```python
from build123d import *

# Parameters (mm, degrees)
F0_W           = 75
F0_H           = 50
F0_R           = 7.6
F1_DEPTH       = 4
F2_D           = 2.4
F3_D           = 3.2
F3_CSINK_D     = 6.72
F3_CSINK_ANGLE = 90
F4_R           = 7.5
F5_R           = 2.5


# Not quite as in the source:
# - a feature names something its author has since deleted; it is built from what else it names


with BuildPart() as f1:
    # F0 (on Top) → F1 (new body)
    with BuildSketch(Plane.XY):
        with Locations((0, 15)):
            Rectangle(F0_W, F0_H)
        Circle(F0_R, mode=Mode.SUBTRACT)
    extrude(amount=-F1_DEPTH)

    # F2 (through all)
    with Locations(Plane.XY):
        with Locations((-8, 8), (8, 8), (8, -8), (-8, -8)):
            Hole(F2_D / 2)

    # F3 (through all)
    with Locations(Plane.XY):
        with Locations((-25, 5), (25, 5), (-5, 28.5), (5, 28.5), (5, 13.5), (-5, 13.5), (-25, 35), (25, 35)):
            CounterSinkHole(F3_D / 2, F3_CSINK_D / 2, counter_sink_angle=F3_CSINK_ANGLE)

    # F4
    f4_edges = [f1.edges().sort_by_distance(p)[0] for p in [
        (-37.5, 40, -2),
        (37.5, 40, -2),
    ]]
    fillet(f4_edges, radius=F4_R)

    # F5
    f5_edges = [f1.edges().sort_by_distance(p)[0] for p in [
        (-37.5, -10, -2),
        (37.5, -10, -2),
    ]]
    fillet(f5_edges, radius=F5_R)


solid = f1.part
```
Can you work these out from the model? Positions are in its coordinate system, mm. Coordinates: 2 decimals unless noted, no trailing zeros. Loops run counter-clockwise (first coordinate to the right, second up) from the corner with the lowest first, then second, coordinate; pieces in that order, holes last. Notation, with made-up numbers: (75.5, 58) -> (119.5, 58) arc R24 ccw to (119.5, 90) -> close; hole circle Ø7 at (15.25, 61). An arc over 180 degrees is marked (long way). Put each result on its own line as item: value. Start each with the question number.
Q1. If I drill on line 1 (Y direction, x = -25, z = -2.55); line 2 (Y direction, x = -8, z = -1.25); line 3 (Y direction, x = -5, z = -2.55), over which ranges is the centre line in solid material (lowest first)? Write a range as [from, to].
Q2. I want a section at C-C (x = 25). Write out the boundary of the cut face in (y, z).
Q3. I want a section at A-A (y = 0). Write out the boundary of the cut face in (x, z).
Q4. I want a section at B-B (z = -2.65). Count the separate pieces of the cut face and the enclosed holes in it, plus the area to 3 significant figures.
Q5. I'm going to push flat-ended pins straight in: P1, Ø1.9, axis at x = 8, y = -8, coming from the +Z side; P2, Ø5, axis at x = -25, y = 35, coming from the +Z side; P3, Ø4, axis at x = 25, y = 35, coming from the +Z side. Where does each tip first touch, or does it pass through?
Q6. I want a section at D-D (y = 28.5). Write out the boundary of the cut face in (x, z).
Q7. Thinking about a two-plate mould opening in Y: for faces 1 (the face through (-35.361, 37.745, -2.028)), 2 (the face through (-4.792, 15.086, -2.896)), 3 (the face through (37.5, 12, -2)), which applies, pulls with the +Y half, pulls with the -Y half, needs draft (parallel to the pull), parting line crosses it, or undercut?
Taken from the geometry:
1. line 1: y = [-10, 3.4], [6.6, 33.4], [36.6, 40]
1. line 2: y = [-10, -9.2], [-6.8, 6.8], [9.2, 40]
1. line 3: y = [-10, -5.72], [5.72, 11.9], [15.1, 26.9], [30.1, 40]
2. outline: (-10, -4) -> (3.4, -4) -> (3.4, -1.76) -> (1.64, 0) -> (-10, 0) -> close; (6.6, -4) -> (33.4, -4) -> (33.4, -1.76) -> (31.64, 0) -> (8.36, 0) -> (6.6, -1.76) -> close; (36.6, -4) -> (40, -4) -> (40, 0) -> (38.36, 0) -> (36.6, -1.76) -> close
3. outline: (-37.5, -4) -> (-7.6, -4) -> (-7.6, 0) -> (-37.5, 0) -> close; (7.6, -4) -> (37.5, -4) -> (37.5, 0) -> (7.6, 0) -> close
4. separate pieces: 1
4. enclosed holes: 13
4. area: 3,460 mm2
5. P1: passes through
5. P2: stops at z = -0.86
5. P3: stops at z = -1.36
6. outline: (-37.5, -4) -> (-6.6, -4) -> (-6.6, -1.76) -> (-8.36, 0) -> (-37.5, 0) -> close; (-3.4, -4) -> (3.4, -4) -> (3.4, -1.76) -> (1.64, 0) -> (-1.64, 0) -> (-3.4, -1.76) -> close; (6.6, -4) -> (37.5, -4) -> (37.5, 0) -> (8.36, 0) -> (6.6, -1.76) -> close
7. face 1: pulls with the +Y half
7. face 2: undercut
7. face 3: needs draft
